Verification items for the finished model (mm, model axes). A direction names the side the tool comes from. Give positions to 0.01 mm unless a question says otherwise; leave off trailing zeros. Order: outer loops, then holes, each group sorted by start corner. A loop starts at its lowest first (then second) coordinate and runs counter-clockwise, first axis right, second up.
from build123d import *

# Parameters (mm, degrees)
SKETCH_1_W           = 37
SKETCH_1_H           = 4.8
SKETCH_1_R           = 0.95
EXTRUDE_1_DEPTH      = 4
EXTRUDE_2_DEPTH      = 21.2
SKETCH_8_W           = 4.5
SKETCH_8_H           = 4.8
EXTRUDE_4_DEPTH      = 8
SKETCH_12_R          = 7.8
CUT_EXTRUDE_3_DEPTH  = 14.5
EXTRUDE_6_DEPTH      = 16.4
EXTRUDE_6_DEPTH_BACK = 4.8
SKETCH_13_W          = 4.5
SKETCH_13_H          = 22
SKETCH_15_R          = 2.5
CUT_EXTRUDE_4_DEPTH  = 14.5
SKETCH_16_W          = 37
SKETCH_16_H          = 4.8
SKETCH_16_R          = 0.95
EXTRUDE_8_DEPTH      = 0.5
SKETCH_19_R          = 0.95
CUT_EXTRUDE_5_DEPTH  = 30
SKETCH_21_W          = 37
SKETCH_21_H          = 0.5
CUT_EXTRUDE_6_DEPTH  = 57.131007474
SKETCH_24_R          = 1
CUT_EXTRUDE_7_DEPTH  = 30
SKETCH_25_R          = 0.95
CUT_EXTRUDE_8_DEPTH  = 10
SKETCH_27_R          = 2
CUT_EXTRUDE_9_DEPTH  = 2


with BuildPart() as part:
    # 草图1 → 凸台-拉伸1 (new body)
    with BuildSketch(Plane.XY):
        with Locations((18.5, -2.4)):
            Rectangle(SKETCH_1_W, SKETCH_1_H)
        with Locations((10, -2.4)):
            Circle(SKETCH_1_R, mode=Mode.SUBTRACT)
        with Locations((27, -2.4)):
            Circle(SKETCH_1_R, mode=Mode.SUBTRACT)
    extrude(amount=EXTRUDE_1_DEPTH)

    # 草图4 → 凸台-拉伸2 (add)
    with BuildSketch(Plane(origin=(0, 0, 0), x_dir=(1, 0, 0), z_dir=(0, 1, 0))):
        Polygon((2.2, 0), (2.2, 4), (5.2, 4), (5.2, 10.5), (2.2, 10.5), (2.2, 14.5), (34.8, 14.5), (34.8, 10.5), (31.8, 10.5), (31.8, 4), (34.8, 4), (34.8, 0), align=None)
    extrude(amount=-EXTRUDE_2_DEPTH)

    # 草图8 → 凸台-拉伸4 (add)
    with BuildSketch(Plane.XY.offset(4)):
        with Locations((18.5, -2.4)):
            Rectangle(SKETCH_8_W, SKETCH_8_H)
    extrude(amount=EXTRUDE_4_DEPTH)

    # 草图12 → 切除-拉伸3 (cut)
    with BuildSketch(Plane.XY):
        with Locations((10, -21.2)):
            Circle(SKETCH_12_R)
        with Locations((27, -21.2)):
            Circle(SKETCH_12_R)
    extrude(amount=-CUT_EXTRUDE_3_DEPTH, mode=Mode.SUBTRACT)

    # 草图13 → 凸台-拉伸6 (add, two sides: drawn at the far end of the back side and taken through both)
    with BuildSketch(Plane.XZ.offset(4.8).offset(-EXTRUDE_6_DEPTH_BACK)):
        with Locations((18.5, 11)):
            Rectangle(SKETCH_13_W, SKETCH_13_H)
    extrude(amount=EXTRUDE_6_DEPTH + EXTRUDE_6_DEPTH_BACK)

    # 草图15 → 切除-拉伸4 (cut)
    with BuildSketch(Plane.XY):
        with Locations((10, -2.4)):
            Circle(SKETCH_15_R)
        with Locations((27, -2.4)):
            Circle(SKETCH_15_R)
    extrude(amount=-CUT_EXTRUDE_4_DEPTH, mode=Mode.SUBTRACT)

    # 草图16 → 凸台-拉伸8 (add)
    with BuildSketch(Plane.XY.offset(4)):
        with Locations((18.5, -2.4)):
            Rectangle(SKETCH_16_W, SKETCH_16_H)
        with Locations((10, -2.4)):
            Circle(SKETCH_16_R, mode=Mode.SUBTRACT)
        with Locations((27, -2.4)):
            Circle(SKETCH_16_R, mode=Mode.SUBTRACT)
    extrude(amount=EXTRUDE_8_DEPTH)

    # 草图19 → 切除-拉伸5 (cut)
    with BuildSketch(Plane.XZ.offset(21.2)):
        with Locations(Location((18.5, 7.5, 0), (0, 0, 270))):
            Circle(SKETCH_19_R)
        with Locations(Location((18.5, 16, 0), (0, 0, 270))):
            Circle(SKETCH_19_R)
    extrude(amount=-CUT_EXTRUDE_5_DEPTH, mode=Mode.SUBTRACT)

    # 草图21 → 切除-拉伸6 (cut, through all)
    with BuildSketch(Plane(origin=(0, 0, -14.5), x_dir=(-1, 0, 0), z_dir=(0, 0, -1))):
        with Locations((-18.5, -0.25)):
            Rectangle(SKETCH_21_W, SKETCH_21_H)
    extrude(amount=-CUT_EXTRUDE_6_DEPTH, mode=Mode.SUBTRACT)

    # 草图24 → 切除-拉伸7 (cut)
    with BuildSketch(Plane(origin=(0, -0.5, 0), x_dir=(1, 0, 0), z_dir=(0, 1, 0))):
        with Locations((18.5, -17)):
            Circle(SKETCH_24_R)
        with Locations((18.5, -7)):
            Circle(SKETCH_24_R)
    extrude(amount=-CUT_EXTRUDE_7_DEPTH, mode=Mode.SUBTRACT)

    # 草图25 → 切除-拉伸8 (cut)
    with BuildSketch(Plane.XZ.offset(4.8)):
        with Locations((5.2, 2.4)):
            Circle(SKETCH_25_R)
        with Locations((31.8, 2.4)):
            Circle(SKETCH_25_R)
    extrude(amount=-CUT_EXTRUDE_8_DEPTH, mode=Mode.SUBTRACT)

    # 草图27 → 切除-拉伸9 (cut)
    with BuildSketch(Plane(origin=(0, -4.8, 0), x_dir=(-1, 0, 0), z_dir=(0, -1, 0))):
        with Locations(Location((-5.2, -2.4, 0), (0, 0, 90))):
            Circle(SKETCH_27_R)
        with Locations(Location((-31.8, -2.4, 0), (0, 0, 90))):
            Circle(SKETCH_27_R)
    extrude(amount=-CUT_EXTRUDE_9_DEPTH, mode=Mode.SUBTRACT)


solid = part.part
(1) Section check A-A, the plane x = 18.5. Enter the section's corners in (y, z).
Solved:
outline: (-21.2, -14.5) - (-0.5, -14.5) - (-0.5, 6) - (-21.2, 6) - close; (-21.2, 8.45) - (-0.5, 8.45) - (-0.5, 15.05) - (-21.2, 15.05) - close; (-21.2, 18) - (-0.5, 18) - (-0.5, 22) - (-21.2, 22) - close
(2) Scan lines: line 1 (Z direction, x = 18.5, y = -16.5); line 2 (X direction, y = -2.4, z = -10); line 3 (Z direction, x = 3, y = -14.25). Record each from-to range of solid material in increasing order.
Solved:
line 1: z = -14.5 to 6, 8.45 to 15.05, 18 to 22
line 2: x = 5.2 to 7.5, 12.5 to 24.5, 29.5 to 31.8
line 3: z = -14.5 to -10.5, -4 to 0
(3) Release check for a two-part mould opening along X. For faces 5 (the flat face through (1, -3, 0)), 6 (the cylindrical face through (6.552, -3.814, 3.874)), 7 (the flat face through (31.8, -8, -7)) record: pulls with the +X half, pulls with the -X half, needs draft (parallel to the pull), parting line crosses it, or undercut.
Solved:
face 5: needs draft
face 6: undercut
face 7: pulls with the +X half
(4) Go/stop test with flat-tipped pins: pin 1 (5 mm diameter, centred on x = 6, z = 1, fed in from -Y); pin 2 (1 mm diameter, centred on x = 27, z = -4, fed in from -Y); pin 3 (1.2 mm diameter, centred on x = 31, z = 2, fed in from -Y). Record where each tip stops, or that it passes through.
Solved:
pin 1: stops at y = -16.59
pin 2: stops at y = -13.42
pin 3: stops at y = -2.8
(5) Section check C-C, the plane y = -18.25. Enter the section's corners in (x, z), then the cut area to 3 significant figures.
Solved:
outline: (2.2, -14.5) - (2.78, -14.5) - (2.78, -10.5) - (2.2, -10.5) - close; (2.2, -4) - (2.78, -4) - (2.78, 0) - (2.2, 0) - close; (16.25, 0) - (17.22, 0) - (17.22, -14.5) - (19.78, -14.5) - (19.78, 0) - (20.75, 0) - (20.75, 22) - (16.25, 22) - close; (34.22, -14.5) - (34.8, -14.5) - (34.8, -10.5) - (34.22, -10.5) - close; (34.22, -4) - (34.8, -4) - (34.8, 0) - (34.22, 0) - close; hole (17.56, 7.35) arc R1 ccw (long way) to (19.44, 7.35) arc R0.95 ccw (long way) to start; hole (17.66, 16.45) arc R0.95 ccw (long way) to (19.34, 16.45) arc R1 ccw (long way) to start
area: 137 mm2
(6) Section check D-D, the plane y = -9. Enter the section's corners in (x, z).
Solved:
outline: (2.2, -14.5) - (34.8, -14.5) - (34.8, -10.5) - (31.8, -10.5) - (31.8, -4) - (34.8, -4) - (34.8, 0) - (20.75, 0) - (20.75, 22) - (16.25, 22) - (16.25, 0) - (2.2, 0) - (2.2, -4) - (5.2, -4) - (5.2, -10.5) - (2.2, -10.5) - close; hole (17.56, 7.35) arc R1 ccw (long way) to (19.44, 7.35) arc R0.95 ccw (long way) to start; hole (17.66, 16.45) arc R0.95 ccw (long way) to (19.34, 16.45) arc R1 ccw (long way) to start
(7) Section check B-B, the plane z = 17. Enter the section's corners in (x, y), then the cut area to 4 significant figures.
Solved:
outline: (16.25, -21.2) - (17.5, -21.2) - (17.5, -0.5) - (16.25, -0.5) - close; (19.5, -21.2) - (20.75, -21.2) - (20.75, -0.5) - (19.5, -0.5) - close
area: 51.75 mm2
(8) Set-up check for faces 1 (the flat face through (4, -8, -4)), 2 (the flat face through (33, -2.8, 2)), 3 (the flat face through (29, -4.8, 2)), 4 (the cylindrical face through (9.9, -4.9, -7.1)): record each of +Z, -Z, +X, -X, +Y, -Y from which the full face is reachable in a straight line by a thin tool's end or side.
Solved:
face 1: -X, +Y, -Y
face 2: -Y
face 3: +Z, +X, -Y
face 4: -Z
